```python
from build123d import *

# Parameters (mm, degrees)
SKETCH_1_W                    = 42
SKETCH_1_H                    = 32
EXTRUDE_1_DEPTH               = 10
SKETCH_2_W                    = 4
SKETCH_2_H                    = 4
CUT_EXTRUDE_1_DEPTH           = 40.56008089
SKETCH_3_W                    = 4
SKETCH_3_H                    = 4
CUT_EXTRUDE_2_DEPTH           = 40.56008089
HOLE_WIZARD_4_0_4_1_D         = 4
HOLE_WIZARD_3_0_3_1_D         = 3
HOLE_WIZARD_3_0_3_1_DEPTH     = 6
HOLE_WIZARD_3_0_3_2_D         = 3
HOLE_WIZARD_3_0_3_2_DEPTH     = 6
HOLE_WIZARD_M20_1_D           = 23
HOLE_WIZARD_M20_1_CBORE_D     = 24
HOLE_WIZARD_M20_1_CBORE_DEPTH = 4
SKETCH_12_R                   = 11.5
SKETCH_12_R_2                 = 9
EXTRUDE_2_DEPTH               = 6
SKETCH_13_R                   = 12
CUT_EXTRUDE_3_DEPTH           = 5
SKETCH_14_R                   = 13
CUT_EXTRUDE_4_DEPTH           = 3


with BuildPart() as part:
    # 草图1 → 凸台-拉伸1 (new body)
    with BuildSketch(Plane.XY.offset(10)):
        Rectangle(SKETCH_1_W, SKETCH_1_H)
    extrude(amount=-EXTRUDE_1_DEPTH)

    # 草图2 → 切除-拉伸1 (cut, through all)
    with BuildSketch(Plane.XZ.offset(16)):
        with Locations((-19, 8)):
            Rectangle(SKETCH_2_W, SKETCH_2_H)
    extrude(amount=-CUT_EXTRUDE_1_DEPTH, mode=Mode.SUBTRACT)

    # 草图3 → 切除-拉伸2 (cut, through all)
    with BuildSketch(Plane.XZ.offset(16)):
        with Locations((19, 8)):
            Rectangle(SKETCH_3_W, SKETCH_3_H)
    extrude(amount=-CUT_EXTRUDE_2_DEPTH, mode=Mode.SUBTRACT)

    # Ø4.0 (4) 直径孔1 (through all)
    with Locations(Plane.XY.offset(10)):
        with Locations((12.374368671, 12.374368671), (12.374368671, -12.374368671), (-12.374368671, -12.374368671), (-12.374368671, 12.374368671)):
            Hole(HOLE_WIZARD_4_0_4_1_D / 2)

    # Ø3.0 (3) 直径孔1
    with Locations(Plane(origin=(21, 0, 0), x_dir=(0, 0, -1), z_dir=(1, 0, 0))):
        with Locations((-3, -10), (-3, 10)):
            Hole(HOLE_WIZARD_3_0_3_1_D / 2, depth=HOLE_WIZARD_3_0_3_1_DEPTH)

    # Ø3.0 (3) 直径孔2
    with Locations(Plane.ZY.offset(21)):
        with Locations((3, -10), (3, 10)):
            Hole(HOLE_WIZARD_3_0_3_2_D / 2, depth=HOLE_WIZARD_3_0_3_2_DEPTH)

    # M20 六角头螺栓的柱形沉头孔1 (through all)
    with Locations(Plane.XY.offset(10)):
        with Locations((0, 0)):
            CounterBoreHole(HOLE_WIZARD_M20_1_D / 2, HOLE_WIZARD_M20_1_CBORE_D / 2, HOLE_WIZARD_M20_1_CBORE_DEPTH)

    # 草图12 → 凸台-拉伸2 (add)
    with BuildSketch(Plane(origin=(0, 0, 0), x_dir=(-1, 0, 0), z_dir=(0, 0, -1))):
        Circle(SKETCH_12_R)
        Circle(SKETCH_12_R_2, mode=Mode.SUBTRACT)
    extrude(amount=-EXTRUDE_2_DEPTH)

    # 草图13 → 切除-拉伸3 (cut)
    with BuildSketch(Plane.XY.offset(10)):
        Circle(SKETCH_13_R)
    extrude(amount=-CUT_EXTRUDE_3_DEPTH, mode=Mode.SUBTRACT)

    # 草图14 → 切除-拉伸4 (cut)
    with BuildSketch(Plane(origin=(0, 0, 0), x_dir=(-1, 0, 0), z_dir=(0, 0, -1))):
        Circle(SKETCH_14_R)
    extrude(amount=-CUT_EXTRUDE_4_DEPTH, mode=Mode.SUBTRACT)


solid = part.part
```
Model file for the job. Use its own axes, mm. A direction names the side the tool comes from. Round coordinates to 2 decimals unless told otherwise and drop trailing zeros. Loops run counter-clockwise (first coordinate to the right, second up) from the corner with the lowest first, then second, coordinate; pieces in that order, holes last. Notation, with made-up numbers: M 41.25,28.25 L 93.25,28.25 A28 cw 93.25,66.25 Z; hole C -11.75,14.5 d6. An arc over 180 degrees is marked long. Put each result on its own line as item: value. Start each with the question number.
Item 1: Cut at C-C (y = 11). Give the number of separate pieces and of enclosed holes in the cut face, then the cut area to 3 significant figures.
Item 2: Cut at D-D (y = 7). List the corners of the cut face in (x, z).
Item 3: Cut at A-A (x = 0). List the corners of the cut face in (y, z), then the cut area to 3 significant figures.
Item 4: Drill centre lines: line 1 along Y through (x, z) = (17.3, 3); line 2 along Y through (x, z) = (-12.5, 8.75); line 3 along Y through (x, z) = (0.5, 2.75). Where is each one in solid material? Low to high.
Item 5: Drop flat-ended pins along their axis: P1, Ø2, axis at y = 11.5, z = 6.5, coming from the -X side; P2, Ø1.2, axis at y = -1, z = 8, coming from the +X side; P3, Ø1.5, axis at y = 9.5, z = 3.5, coming from the +X side; P4, Ø3, axis at x = 19, y = 4, coming from the +Z side. Give the stop position or say it passes through.
Item 6: 3-axis set-ups, long thin cutter, end or side, ignore diameter. For faces 1 (the face through (-19, 0, 6)), 2 (the face through (17, 0, 8)), 3 (the face through (-15, 10, 3)), 4 (the face through (-11.99, 0.53, 7.54)): which of +Z, -Z, +X, -X, +Y, -Y reach the whole face in a straight line?
Item 7: Mould opens along Z. For faces 5 (the face through (-17.958, 9.425, 1.614)), 6 (the face through (21, 0, 3)), 7 (the face through (2, 9, 5)) say: released by +Z, released by -Z, zero draft, split by the parting line, or undercut.
Item 8: Cut at B-B (y = 0). List the corners of the cut face in (x, z).
Answer block:
1. separate pieces: 3
1. enclosed holes: 0
1. area: 214 mm2
2. outline: M -21,0 L -10.95,0 L -10.95,3 L -5.66,3 L -5.66,5 L -9.75,5 L -9.75,10 L -17,10 L -17,6 L -21,6 Z; M 5.66,3 L 10.95,3 L 10.95,0 L 21,0 L 21,6 L 17,6 L 17,10 L 9.75,10 L 9.75,5 L 5.66,5 Z
3. outline: M -16,0 L -13,0 L -13,3 L -9,3 L -9,5 L -12,5 L -12,10 L -16,10 Z; M 9,3 L 13,3 L 13,0 L 16,0 L 16,10 L 12,10 L 12,5 L 9,5 Z
3. area: 86.0 mm2
4. line 1: -16 to -11.5, -8.5 to 8.5, 11.5 to 16
4. line 2: -16 to -14.37, -10.38 to 10.38, 14.37 to 16
4. line 3: -16 to -12.99, 12.99 to 16
5. P1: x = -21
5. P2: x = 17
5. P3: x = 15
5. P4: z = 6
6. face 1: +Z, -X, +Y, -Y
6. face 2: +Z, +X, +Y, -Y
6. face 3: -X
6. face 4: +Z
7. face 5: undercut
7. face 6: zero draft
7. face 7: released by +Z
8. outline: M -21,0 L -13,0 L -13,3 L -9,3 L -9,5 L -12,5 L -12,10 L -17,10 L -17,6 L -21,6 Z; M 9,3 L 13,3 L 13,0 L 21,0 L 21,6 L 17,6 L 17,10 L 12,10 L 12,5 L 9,5 Z
